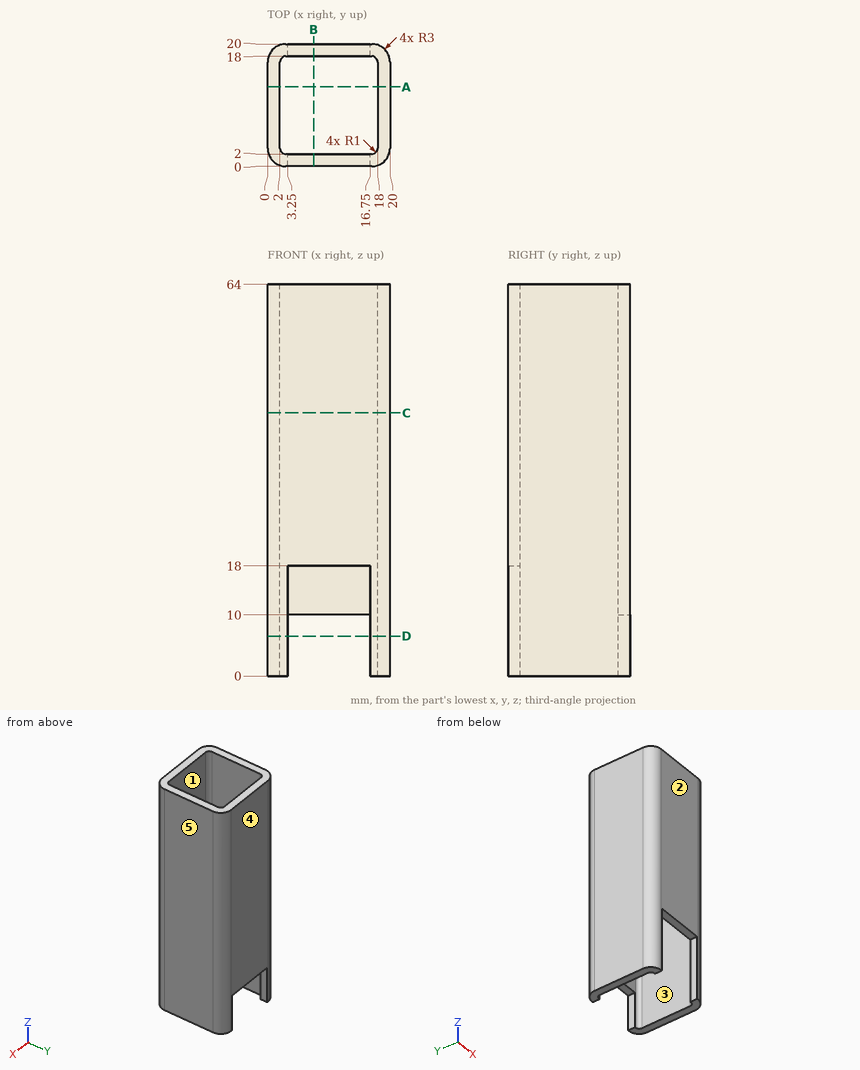
Study the drawing (mm; zero at the part's minimum x, y, z) and answer. A direction names the side the tool comes from. Coordinates: 2 decimals unless noted, no trailing zeros. Order: outer loops, then holes, each group sorted by start corner. A loop starts at its lowest first (then second) coordinate and runs counter-clockwise, first axis right, second up. Notation, with made-up numbers: M 31,69.25 L 42,69.25 A31 cw 42,97.25 Z; hole C 29.25,-15 d4. An arc over 180 degrees is marked long. Use CSV: the item, a comma, the result in double quotes.
Q1. Section B-B (x = 7.5) is taken. Determine the outline of the cut face in (y, z).
Here are the results:
outline,"M 0,18 L 2,18 L 2,64 L 0,64 Z; M 18,10 L 20,10 L 20,64 L 18,64 Z"
Q2. Straight lines are drawn through the part: L1, parallel to X at y = 11.5, z = 4.5; L2, parallel to Y at x = 17.75, z = 22. For each, find the intervals that lie inside material, in ascending order.
Here are the results:
L1,"0 to 2, 18 to 20"
L2,"0.1 to 2.34, 17.66 to 19.9"
Q3. Section D-D (z = 6.5) is taken. Determine the outline of the cut face in (x, y).
Here are the results:
outline,"M 0,3 A3 ccw 3,0 L 3.25,0 L 3.25,2 L 3,2 A1 cw 2,3 L 2,17 A1 cw 3,18 L 3.25,18 L 3.25,20 L 3,20 A3 ccw 0,17 Z; M 16.75,0 L 17,0 A3 ccw 20,3 L 20,17 A3 ccw 17,20 L 16.75,20 L 16.75,18 L 17,18 A1 cw 18,17 L 18,3 A1 cw 17,2 L 16.75,2 Z"
Q4. Given pin 1 Ø2 at (y, z) = (19, 5) entering from -X; pin 2 Ø1 at (y, z) = (0.5, 8.5) entering from -X; pin 3 Ø1.6 at (y, z) = (1, 8) entering from +X, each flat-ended and moving along its own axis, determine where each tip first touches the part or whether it passes through.
Here are the results:
pin 1,"x = 0.17"
pin 2,"x = 0.76"
pin 3,"x = 19.75"
Q5. Section A-A (y = 13) is taken. Determine the outline of the cut face in (x, z), then the cut area to 3 significant figures.
Here are the results:
outline,"M 0,0 L 2,0 L 2,64 L 0,64 Z; M 18,0 L 20,0 L 20,64 L 18,64 Z"
area,"256 mm2"
Q6. A tool of negligible diameter and unlimited length cuts with its end or side. For the marked faces 1 and 2, from which of +Z, -Z, +X, -X, +Y, -Y can it reach the whole face along a straight path? Write none if from no direction.
Here are the results:
face 1,"+Z, -Z"
face 2,"+Z, -Z, +X, -X, -Y"
Q7. Section C-C (z = 43) is taken. Determine the outline of the cut face in (x, y).
Here are the results:
outline,"M 0,3 A3 ccw 3,0 L 17,0 A3 ccw 20,3 L 20,17 A3 ccw 17,20 L 3,20 A3 ccw 0,17 Z; hole M 2,3 A1 ccw 3,2 L 17,2 A1 ccw 18,3 L 18,17 A1 ccw 17,18 L 3,18 A1 ccw 2,17 Z"
Q8. Determine the mould class of the marked faces 3, 4 and 5 for opening direction Y: pulls with the +Y half, pulls with the -Y half, needs draft (parallel to the pull), parting line crosses it, or undercut.
Here are the results:
face 3,"undercut"
face 4,"pulls with the +Y half"
face 5,"needs draft"
